The listing builds one solid part. Answer for the finished solid, in the listing's coordinates (mm). A direction names the side the tool comes from. Round coordinates to 2 decimals unless told otherwise and drop trailing zeros. Write each loop counter-clockwise with the first axis right and the second up, starting at its lowest first coordinate (ties: lowest second). Pieces come first, ordered by that corner, then holes. Notation, with made-up numbers: (67.25, 50.25) - (97.25, 50.25) arc R18 cw to (97.25, 56.25) - close; hole circle Ø8 at (-5, 6.25). An arc over 180 degrees is marked (long way). Return JSON: item names as keys, results as strings. Group by question number.
Autodesk Inventor part; units mm, degrees
ref_plane "YZ Plane" through (0, 0, 0) normal (1, 0, 0) x (0, 1, 0)
ref_plane "XZ Plane" through (0, 0, 0) normal (0, 1, 0) x (-1, 0, 0)
ref_plane "XY Plane" through (0, 0, 0) normal (0, 0, 1) x (1, 0, 0)
sketch "Boceto1" plane through (0, 0, 0) normal (0, 1, 0) x (-1, 0, 0)
  line L0 (6.207, 40.007) -> (6.207, 26.007)
  line L1 (6.207, 26.007) -> (-56.793, 26.007)
  line L2 (-56.793, 26.007) -> (-56.793, 40.007)
  line L3 (-56.793, 40.007) -> (6.207, 40.007)
  circle A0 centre (-25.293, 31.257) radius 2
  circle A1 centre (-2.543, 31.257) radius 2
  circle A2 centre (-48.043, 31.257) radius 2
  point P0 (0, 0)
  point P1 (0, 0)
  dimension "d0" = 14
  dimension "d1" = 63
  dimension "d24" = 4
  dimension "d25" = 4
  dimension "d26" = 4
  dimension "d27" = 8.75
  dimension "d28" = 8.75
  dimension "d29" = 8.75
  dimension "d30" = 31.5
  dimension "d31" = 8.75
  dimension "d32" = 8.75
extrude "Extrusión1" add sketch "Boceto1" along normal blind 0.8
sketch "Boceto7" plane through (56.793, 0, 40.007) normal (1, 0, 0) x (0, 0, -1)
  circle A0 centre (16.375, -1.575) radius 2.375
  circle A1 centre (16.375, -1.575) radius 1.625
  line L0 (0, 0.8) -> (14, 0.8)
  line L1 (14, 0) -> (14, 0.8)
  line L2 (14, 0) -> (14, -1.575)
  line L3 (16.375, 0.8) -> (14, 0.8)
  line L4 (14, 0) -> (0, 0)
  line L5 (14, 0.8) -> (14, 0)
  point P0 (40.007, 0)
  dimension "d33" = 4.75
  dimension "d34" = 3.25
extrude "Extrusión6" add sketch "Boceto7" against normal blind 44.5
sketch "Boceto9" plane through (56.793, 0, 40.007) normal (1, 0, 0) x (0, 0, -1)
  circle A0 centre (16.375, -1.575) radius 1.625
  circle A1 centre (16.375, -1.575) radius 2.375
  line L0 (14, 0.8) -> (16.375, 0.8)
  line L1 (16.375, 0.8) -> (14, 0.8)
  line L2 (14, -1.575) -> (14, 0)
  line L3 (14, 0.8) -> (14, -1.575)
  point P0 (40.007, 0)
extrude "Extrusión8" cut sketch "Boceto9" against normal blind 18.5 contours A0 | A1 | A1 L2 L3 L0
properties part number "Ala 2 Bisagra tipo Libro Chica"
(1) Flat-ended cylindrical pins translate along their axes: pin 1 (1.4 mm diameter, centred on y = -2.5, z = 24.5, fed in from -X); pin 2 (1.7 mm diameter, centred on x = 26, y = -1, fed in from +Z); pin 3 (4 mm diameter, centred on x = 19.5, z = 34, fed in from -Y); pin 4 (3 mm diameter, centred on x = 48.043, z = 31.257, fed in from +Y). Find the tip coordinate at first contact, or state that the pin passes through.
(2) Find section B-B (z = 22.75). Write down the section's boundary in (x, y), plus the area to 3 significant figures.
(3) Find section A-A (x = 28). Write down the section's boundary in (y, z) (3 decimals).
(4) Find section C-C (y = -2.5). Write down the section's boundary in (x, z).
(5) Consider line 1 (Z direction, x = 24, y = -1.7); line 2 (Y direction, x = 28, z = 32.5); line 3 (Z direction, x = 20.5, y = -0.6). Determine where each line is inside the solid, lowest interval first.
(6) For faces 4 (the cylindrical face through (2.803, 0.394, 29.274)), 5 (the flat face through (38.293, 0, 25)), 6 (the flat face through (26, 0, 35)), determine the directions among +Z, -Z, +X, -X, +Y, -Y from which every point of the face is accessible in a straight line to the end or side of a thin tool.
(7) Determine the mould class of faces 1 (the cylindrical face through (25.475, -1.504, 25.255)), 2 (the flat face through (25, -1, 26.007)), 3 (the flat face through (12.293, 0, 25)) for opening direction Z: +Z half, -Z half, draft (parallel to the pull), parting line (faces both ways), or undercut.
(8) Find section D-D (z = 38). Write down the section's boundary in (x, y).
Check sheet entries:
{
 "1": {"pin 1": "stops at x = 12.29", "pin 2": "stops at z = 26.01", "pin 3": "stops at y = 0", "pin 4": "passes through"},
 "2": {"outline": "(12.29, -3.78) - (38.29, -3.78) - (38.29, -2.94) - (12.29, -2.94) - close; (12.29, -0.21) - (38.29, -0.21) - (38.29, 0.63) - (12.29, 0.63) - close", "area": "43.7 mm^2"},
 "3": {"outline": "(-1.575, 26.007) arc R2.375 ccw (long way) to (0.8, 23.632) - (0.8, 40.007) - (0, 40.007) - (0, 26.007) - close; hole circle Ø3.25 at (-1.575, 23.632)"},
 "4": {"outline": "(12.29, 21.44) - (38.29, 21.44) - (38.29, 22.3) - (12.29, 22.3) - close; (12.29, 24.97) - (38.29, 24.97) - (38.29, 25.82) - (12.29, 25.82) - close"},
 "5": {"line 1": "z = 21.26 to 22.01, 25.25 to 26", "line 2": "y = 0 to 0.8", "line 3": "z = 21.47 to 22.33, 24.93 to 26.01"},
 "6": {"face 4": "+Y, -Y", "face 5": "-Z, +X, +Y, -Y", "face 6": "+Z, +X, -X, -Y"},
 "7": {"face 1": "undercut", "face 2": "+Z half", "face 3": "draft"},
 "8": {"outline": "(-6.21, 0) - (56.79, 0) - (56.79, 0.8) - (-6.21, 0.8) - close"}
}
